from build123d import *

# Parameters (mm, degrees)
F1_DEPTH = 32


# Not quite as in the source:
# - a feature names something its author has since deleted; it is built from what else it names


with BuildPart() as f1:
    # F0 (on Front) → F1 (new body)
    with BuildSketch(Plane.XZ):
        with BuildLine():
            Line((0.200491711, 11.3311297744), (-6.6555393256, 10.8363182701))
            Line((-6.6555393256, 10.8363182701), (-0.9784149812, 10.8363182701))
            ThreePointArc((-0.9784149812, 10.8363182701), (-0.429566386, 11.1804663417), (0.200491711, 11.3311297744))
        make_face()
        with BuildLine():
            Line((-0.9784149812, 10.8363182701), (-6.6555393256, 10.8363182701))
            Line((-6.6555393256, 10.8363182701), (-6.6555393256, 9.8363182701))
            Line((-6.6555393256, 9.8363182701), (-1.5920309988, 9.8363182701))
            ThreePointArc((-1.5920309988, 9.8363182701), (-1.3602002438, 10.382325514), (-0.9784149812, 10.8363182701))
        make_face()
        with BuildLine():
            ThreePointArc((0.200491711, 11.3311297744), (-0.429566386, 11.1804663417), (-0.9784149812, 10.8363182701))
            Line((-0.9784149812, 10.8363182701), (0.3444606744, 10.8363182701))
            Line((0.3444606744, 10.8363182701), (1.6673363299, 10.8363182701))
            ThreePointArc((1.6673363299, 10.8363182701), (0.9837296736, 11.2314001012), (0.200491711, 11.3311297744))
        make_face()
        with BuildLine():
            Line((0.3444606744, 10.8363182701), (-0.9784149812, 10.8363182701))
            ThreePointArc((-0.9784149812, 10.8363182701), (-1.3602002438, 10.382325514), (-1.5920309988, 9.8363182701))
            Line((-1.5920309988, 9.8363182701), (-1.069752888, 9.8363182701))
            ThreePointArc((-1.069752888, 9.8363182701), (-0.5215647294, 10.5610631415), (0.3444606744, 10.8363182701))
        make_face()
        with BuildLine():
            Line((1.6673363299, 10.8363182701), (0.3444606744, 10.8363182701))
            ThreePointArc((0.3444606744, 10.8363182701), (1.4051208461, 10.3969784419), (1.8444606744, 9.3363182701))
            ThreePointArc((1.8444606744, 9.3363182701), (1.4051208461, 8.2756580983), (0.3444606744, 7.8363182701))
            Line((0.3444606744, 7.8363182701), (1.6673363299, 7.8363182701))
            ThreePointArc((1.6673363299, 7.8363182701), (2.1673363299, 8.5134426146), (2.3444606744, 9.3363182701))
            ThreePointArc((2.3444606744, 9.3363182701), (2.1673363299, 10.1591939256), (1.6673363299, 10.8363182701))
        make_face()
        with BuildLine():
            Line((-1.5920309988, 8.8363182701), (-6.6555393256, 8.8363182701))
            Line((-6.6555393256, 8.8363182701), (-6.6555393256, 7.8363182701))
            Line((-6.6555393256, 7.8363182701), (-0.9784149812, 7.8363182701))
            ThreePointArc((-0.9784149812, 7.8363182701), (-1.3602002438, 8.2903110262), (-1.5920309988, 8.8363182701))
        make_face()
        with BuildLine():
            Line((5.0215850188, 10.8363182701), (1.6673363299, 10.8363182701))
            ThreePointArc((1.6673363299, 10.8363182701), (2.1673363299, 10.1591939256), (2.3444606744, 9.3363182701))
            ThreePointArc((2.3444606744, 9.3363182701), (2.1673363299, 8.5134426146), (1.6673363299, 7.8363182701))
            Line((1.6673363299, 7.8363182701), (5.0215850188, 7.8363182701))
            ThreePointArc((5.0215850188, 7.8363182701), (4.3444606744, 9.3363182701), (5.0215850188, 10.8363182701))
        make_face()
        with BuildLine():
            Line((-1.069752888, 8.8363182701), (-1.5920309988, 8.8363182701))
            ThreePointArc((-1.5920309988, 8.8363182701), (-1.3602002438, 8.2903110262), (-0.9784149812, 7.8363182701))
            Line((-0.9784149812, 7.8363182701), (0.3444606744, 7.8363182701))
            ThreePointArc((0.3444606744, 7.8363182701), (-0.5215647294, 8.1115733987), (-1.069752888, 8.8363182701))
        make_face()
        with BuildLine():
            Line((-0.9784149812, 7.8363182701), (-6.6555393256, 7.8363182701))
            Line((-6.6555393256, 7.8363182701), (0.200491711, 7.3415067658))
            ThreePointArc((0.200491711, 7.3415067658), (-0.429566386, 7.4921701986), (-0.9784149812, 7.8363182701))
        make_face()
        with BuildLine():
            ThreePointArc((6.4884296377, 11.3311297744), (5.7051916751, 11.2314001012), (5.0215850188, 10.8363182701))
            Line((5.0215850188, 10.8363182701), (6.344460699, 10.8363182701))
            Line((6.344460699, 10.8363182701), (7.6673363299, 10.8363182701))
            ThreePointArc((7.6673363299, 10.8363182701), (7.1184877347, 11.1804663417), (6.4884296377, 11.3311297744))
        make_face()
        with BuildLine():
            Line((6.344460699, 10.8363182701), (5.0215850188, 10.8363182701))
            ThreePointArc((5.0215850188, 10.8363182701), (4.3444606744, 9.3363182701), (5.0215850188, 7.8363182701))
            Line((5.0215850188, 7.8363182701), (6.3444606473, 7.8363182701))
            ThreePointArc((6.3444606473, 7.8363182701), (4.8444606744, 9.336318296), (6.344460699, 10.8363182701))
        make_face()
        with BuildLine():
            Line((1.6673363299, 7.8363182701), (0.3444606744, 7.8363182701))
            Line((0.3444606744, 7.8363182701), (-0.9784149812, 7.8363182701))
            ThreePointArc((-0.9784149812, 7.8363182701), (-0.429566386, 7.4921701986), (0.200491711, 7.3415067658))
            ThreePointArc((0.200491711, 7.3415067658), (0.9837296736, 7.441236439), (1.6673363299, 7.8363182701))
        make_face()
        with BuildLine():
            Line((7.6673363299, 10.8363182701), (6.344460699, 10.8363182701))
            ThreePointArc((6.344460699, 10.8363182701), (7.2104860882, 10.5610631344), (7.7586742367, 9.8363182701))
            Line((7.7586742367, 9.8363182701), (8.2809523475, 9.8363182701))
            ThreePointArc((8.2809523475, 9.8363182701), (8.0491215925, 10.382325514), (7.6673363299, 10.8363182701))
        make_face()
        with BuildLine():
            Line((13.3444606744, 10.8363182701), (6.4884296377, 11.3311297744))
            ThreePointArc((6.4884296377, 11.3311297744), (7.1184877347, 11.1804663417), (7.6673363299, 10.8363182701))
            Line((7.6673363299, 10.8363182701), (13.3444606744, 10.8363182701))
        make_face()
        with BuildLine():
            Line((6.3444606473, 7.8363182701), (5.0215850188, 7.8363182701))
            ThreePointArc((5.0215850188, 7.8363182701), (5.7051916751, 7.441236439), (6.4884296377, 7.3415067658))
            ThreePointArc((6.4884296377, 7.3415067658), (7.1184877347, 7.4921701986), (7.6673363299, 7.8363182701))
            Line((7.6673363299, 7.8363182701), (6.3444606473, 7.8363182701))
        make_face()
        with BuildLine():
            Line((13.3444606744, 10.8363182701), (7.6673363299, 10.8363182701))
            ThreePointArc((7.6673363299, 10.8363182701), (8.0491215925, 10.382325514), (8.2809523475, 9.8363182701))
            Line((8.2809523475, 9.8363182701), (13.3444606744, 9.8363182701))
            Line((13.3444606744, 9.8363182701), (13.3444606744, 10.8363182701))
        make_face()
        with BuildLine():
            ThreePointArc((7.7586742367, 8.8363182701), (7.2104860671, 8.1115733909), (6.3444606473, 7.8363182701))
            Line((6.3444606473, 7.8363182701), (7.6673363299, 7.8363182701))
            ThreePointArc((7.6673363299, 7.8363182701), (8.0491215925, 8.2903110262), (8.2809523475, 8.8363182701))
            Line((8.2809523475, 8.8363182701), (7.7586742367, 8.8363182701))
        make_face()
        with BuildLine():
            ThreePointArc((7.6673363299, 7.8363182701), (7.1184877347, 7.4921701986), (6.4884296377, 7.3415067658))
            Line((6.4884296377, 7.3415067658), (13.3444606744, 7.8363182701))
            Line((13.3444606744, 7.8363182701), (7.6673363299, 7.8363182701))
        make_face()
        with BuildLine():
            ThreePointArc((8.2809523475, 8.8363182701), (8.0491215925, 8.2903110262), (7.6673363299, 7.8363182701))
            Line((7.6673363299, 7.8363182701), (13.3444606744, 7.8363182701))
            Line((13.3444606744, 7.8363182701), (13.3444606744, 8.8363182701))
            Line((13.3444606744, 8.8363182701), (8.2809523475, 8.8363182701))
        make_face()
    extrude(amount=F1_DEPTH)


solid = f1.part
Source: CAD feature listing. Evaluate the final solid. Frame: model axes, mm. A direction names the side the tool comes from. Coordinates: 2 decimals unless noted, no trailing zeros. Loops run counter-clockwise (first coordinate to the right, second up) from the corner with the lowest first, then second, coordinate; pieces in that order, holes last. Notation, with made-up numbers: (-37.5, 52) - (1.5, 52) arc R11 ccw to (1.5, 69) - close; hole circle Ø5 at (-10, 79). An arc over 180 degrees is marked (long way). Return JSON: item names as keys, results as strings.
Q1. Mould query, pull axis X, two halves, no side actions, for faces 6 (the flat face through (3, -16, 7.836)), 7 (the cylindrical face through (5.695, -15.776, 7.445)), 8 (the flat face through (-6.656, -16, 10)), 9 (the flat face through (9.96, -15.78, 11.08)). Classes: released by +X, released by -X, zero draft, split by the parting line, or undercut.
Results:
{"face 6": "undercut", "face 7": "undercut", "face 8": "released by -X", "face 9": "released by +X"}
Q2. Material intervals for line 1 along X through (y, z) = (-9, 8.05); line 2 along X through (y, z) = (-27.5, 8.2); line 3 along Z through (x, y) = (3.5, -15), sorted ascending.
Results:
{"line 1": "-6.66 to -0.43, 1.12 to 5.57, 7.12 to 13.34", "line 2": "-6.66 to -0.63, 1.32 to 5.37, 7.32 to 13.34", "line 3": "7.84 to 10.84"}
Q3. Contact query for flat-ended pins moving along their axis: P1, Ø6, axis at x = -3.5, y = -12.5, coming from the -Z side; P2, Ø6, axis at x = 11, y = -23, coming from the +Z side; P3, Ø4, axis at x = 1, y = -24, coming from the +Z side; P4, Ø1.7, axis at x = 3.5, y = -13, coming from the -Z side. Output: stop coordinate, or through.
Results:
{"P1": "z = 7.39", "P2": "z = 11.22", "P3": "z = 11.34", "P4": "z = 7.84"}
Q4. Section A-A, the plane x = 9.75. Return loops of the section in (y, z).
Results:
{"outline": "(-32, 7.58) - (0, 7.58) - (0, 8.84) - (-32, 8.84) - close; (-32, 9.84) - (0, 9.84) - (0, 11.1) - (-32, 11.1) - close"}
Q5. Section C-C, the plane z = 10.5. Return loops of the section in (x, y).
Results:
{"outline": "(-6.66, -32) - (-0.6, -32) - (-0.6, 0) - (-6.66, 0) - close; (1.29, -32) - (5.4, -32) - (5.4, 0) - (1.29, 0) - close; (7.29, -32) - (13.34, -32) - (13.34, 0) - (7.29, 0) - close"}
Q6. Section B-B, the plane y = -18.5. Return loops of the section in (x, z), plus the area to 3 significant figures.
Results:
{"outline": "(-6.66, 7.84) - (0.2, 7.34) arc R2 ccw to (1.67, 7.84) - (5.02, 7.84) arc R2 ccw to (6.49, 7.34) - (13.34, 7.84) - (13.34, 8.84) - (7.76, 8.84) arc R1.5 cw (long way) to (7.76, 9.84) - (13.34, 9.84) - (13.34, 10.84) - (6.49, 11.33) arc R2 ccw to (5.02, 10.84) - (1.67, 10.84) arc R2 ccw to (0.2, 11.33) - (-6.66, 10.84) - (-6.66, 9.84) - (-1.07, 9.84) arc R1.5 cw (long way) to (-1.07, 8.84) - (-6.66, 8.84) - close", "area": "43.7 mm2"}
Q7. Access query for faces 1 (the flat face through (3, -16, 10.836)), 2 (the flat face through (11, -16, 9.836)), 3 (the flat face through (13.344, -16, 8)), 4 (the flat face through (-4, -16, 8.836)), 5 (the flat face through (9.868, -15.776, 7.585)). Directions: +Z, -Z, +X, -X, +Y, -Y. A direction counts if a zero-diameter tool reaches every point of the face in a straight line with its end or side. Return the directions, or none.
Results:
{"face 1": "+Z, +Y, -Y", "face 2": "+X, +Y, -Y", "face 3": "+Z, -Z, +X, +Y, -Y", "face 4": "-X, +Y, -Y", "face 5": "-Z, +X, +Y, -Y"}
Q8. Section D-D, the plane x = 3.75. Return loops of the section in (y, z), plus the area to 3 significant figures.
Results:
{"outline": "(-32, 7.84) - (0, 7.84) - (0, 10.84) - (-32, 10.84) - close", "area": "96.0 mm2"}
